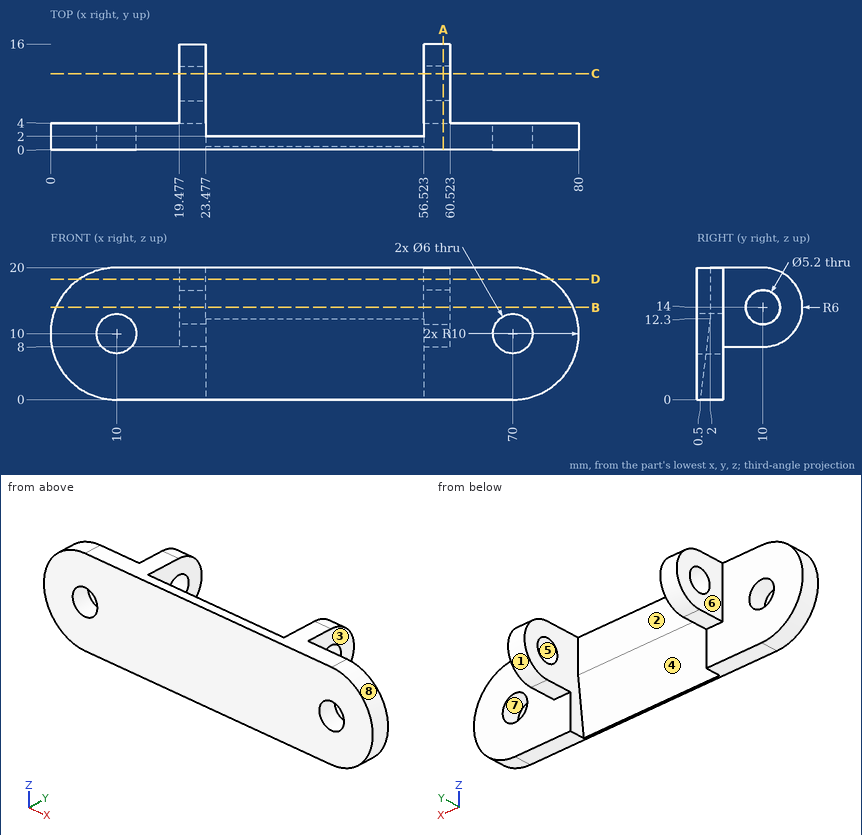
Can you work these out from the drawing? Everything is in mm from the part's minimum corner. A direction names the side the tool comes from. Coordinates: 2 decimals unless noted, no trailing zeros. Loops run counter-clockwise (first coordinate to the right, second up) from the corner with the lowest first, then second, coordinate; pieces in that order, holes last.
1. If we mould it in two halves opening along X, with no side actions, what happens to the marked faces 6, 7 and 8? For each: pulls with the +X half, pulls with the -X half, needs draft (parallel to the pull), parting line crosses it, or undercut.
2. Imagine slicing it at C-C, the plane y = 11.5. Please give me the cut outline in (x, z).
3. For the marked faces 1, 2, 3, 4 and 5, which set-ups out of +Z, -Z, +X, -X, +Y, -Y let a thin tool reach every point of the face, with its end or its side?
4. Imagine slicing it at B-B, the plane z = 14. Please give me the cut outline in (x, y) (1 decimal).
5. Imagine slicing it at D-D, the plane z = 18.25. Please give me the cut outline in (x, y) (1 decimal).
6. I need wall thicknesses on L1, parallel to X at y = 2.95, z = 10; L2, parallel to X at y = 1.25, z = 10; L3, parallel to Y at x = 22.5, z = 13.75 (1 decimal). Which ranges of each line are inside material? Lowest first, please.
7. For P1, Ø6, axis at x = 44, z = 14.5, coming from the +Y side; P2, Ø7, axis at y = 10, z = 14, coming from the -X side; P3, Ø1.5, axis at x = 11.5, y = 6, coming from the +Z side; P4, Ø2, axis at x = 15, z = 9.5, coming from the +Y side, each with a flat end and sliding along its axis, tell me the tip position at first contact or that it passes through.
8. Imagine slicing it at A-A, the plane x = 59.5. Please give me the cut outline in (y, z).
Taken from the geometry:
1. face 6: pulls with the -X half
1. face 7: undercut
1. face 8: pulls with the +X half
2. outline: (19.48, 8.19) - (23.48, 8.19) - (23.48, 11.88) - (19.48, 11.88) - close; (19.48, 16.12) - (23.48, 16.12) - (23.48, 19.81) - (19.48, 19.81) - close; (56.52, 8.19) - (60.52, 8.19) - (60.52, 11.88) - (56.52, 11.88) - close; (56.52, 16.12) - (60.52, 16.12) - (60.52, 19.81) - (56.52, 19.81) - close
3. face 1: +X, -X, +Y
3. face 2: +Z, -Z, +Y
3. face 3: +Z, -Z, +X, +Y
3. face 4: -Z, +Y
3. face 5: +X, -X
4. outline: (0.8, 0) - (79.2, 0) - (79.2, 4) - (60.5, 4) - (60.5, 7.4) - (56.5, 7.4) - (56.5, 2) - (23.5, 2) - (23.5, 7.4) - (19.5, 7.4) - (19.5, 4) - (0.8, 4) - close; (19.5, 12.6) - (23.5, 12.6) - (23.5, 16) - (19.5, 16) - close; (56.5, 12.6) - (60.5, 12.6) - (60.5, 16) - (56.5, 16) - close
5. outline: (4.3, 0) - (75.7, 0) - (75.7, 4) - (60.5, 4) - (60.5, 14.2) - (56.5, 14.2) - (56.5, 2) - (23.5, 2) - (23.5, 14.2) - (19.5, 14.2) - (19.5, 4) - (4.3, 4) - close
6. L1: x = 0 to 7, 13 to 23.48, 56.52 to 67, 73 to 80
6. L2: x = 0 to 7, 13 to 67, 73 to 80
6. L3: y = 0 to 7.4, 12.6 to 16
7. P1: stops at y = 2
7. P2: stops at x = 19.48
7. P3: passes through
7. P4: stops at y = 4
8. outline: (0, 0) - (4, 0) - (4, 8) - (10, 8) arc R6 ccw to (10, 20) - (0, 20) - close; hole circle Ø5.2 at (10, 14)
